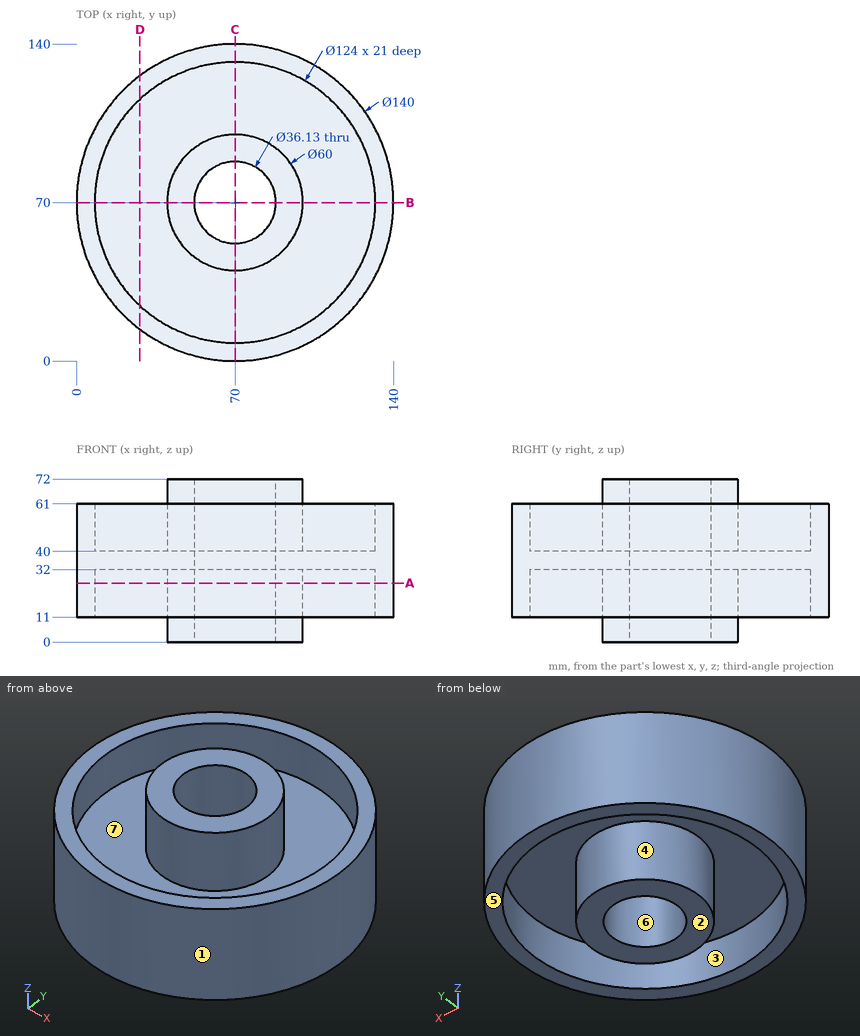
Geometry: see drawing. Coordinates: mm, zero at the bounding-box minimum. A direction names the side the tool comes from. Give positions to 0.01 mm unless a question says otherwise; leave off trailing zeros. Loops run counter-clockwise (first coordinate to the right, second up) from the corner with the lowest first, then second, coordinate; pieces in that order, holes last. Notation, with made-up numbers: M 59,47 L 94,47 A24 ccw 94,78 Z; hole C 62,-27.5 d4. An arc over 180 degrees is marked long. Use one line per item in the form item = value.
1. Section query D-D, the plane x = 28. Return the cut outline in (y, z), and give its area (3 significant figures).
Numbers:
outline = M 14,11 L 24.39,11 L 24.39,32 L 115.61,32 L 115.61,11 L 126,11 L 126,61 L 115.61,61 L 115.61,40 L 24.39,40 L 24.39,61 L 14,61 Z
area = 1,770 mm²
2. First-contact query: pin 1 (8 mm diameter, centred on y = 62.5, z = 18, fed in from -X); pin 2 (1.5 mm diameter, centred on y = 65.5, z = 53.5, fed in from +X); pin 3 (4 mm diameter, centred on x = 73.5, z = 38, fed in from +Y). Flat tips, straight axial feed; report the tip coordinate or a pass-through.
Numbers:
pin_1 = 0.09
pin_2 = 139.9
pin_3 = 139.98
3. Pull-direction query (X, two-part tool) for the marked faces 1, 2, 3 and 4; classes: released by +X, released by -X, zero draft, split by the parting line, or undercut.
Numbers:
face_1 = split by the parting line
face_2 = zero draft
face_3 = undercut
face_4 = undercut
4. Section query A-A, the plane z = 26. Return the cut outline in (x, y) (3 decimals).
Numbers:
outline = C 70,70 d140; C 70,70 d60; hole C 70,70 d124; hole C 70,70 d36.13
5. Section query B-B, the plane y = 70. Return the cut outline in (x, z) (3 decimals), and give its area (3 significant figures).
Numbers:
outline = M 0,11 L 8,11 L 8,32 L 40,32 L 40,0 L 51.935,0 L 51.935,72 L 40,72 L 40,40 L 8,40 L 8,61 L 0,61 Z; M 88.065,0 L 100,0 L 100,32 L 132,32 L 132,11 L 140,11 L 140,61 L 132,61 L 132,40 L 100,40 L 100,72 L 88.065,72 Z
area = 3,030 mm²
6. Line query: L1, parallel to Y at x = 70, z = 48 (3 decimals); L2, parallel to X at y = 81, z = 27; L3, parallel to Y at x = 78, z = 16. Output: solid intervals per line, ascending.
Numbers:
L1 = 0 to 8, 40 to 51.935, 88.065 to 100, 132 to 140
L2 = 0.87 to 8.98, 42.09 to 55.67, 84.33 to 97.91, 131.02 to 139.13
L3 = 0.46 to 8.52, 41.09 to 53.8, 86.2 to 98.91, 131.48 to 139.54
7. Reachability of the marked faces 5, 6 and 7 from +Z, -Z, +X, -X, +Y, -Y: full face, straight path, thin tool, end or side. Return the list, or none.
Numbers:
face_5 = -Z
face_6 = +Z, -Z
face_7 = +Z
